```python
from build123d import *

# Parameters (mm, degrees)
SKETCH_1_W          = 25
SKETCH_1_H          = 20
EXTRUDE_1_DEPTH     = 10
EXTRUDE_2_DEPTH     = 10
SKETCH_3_W          = 10
SKETCH_3_H          = 10
CUT_EXTRUDE_1_DEPTH = 15
FILLET_1_DEPTH      = 10
FILLET_START        = -1
FILLET_1_2_DEPTH    = 6
FILLET_1_3_DEPTH    = 6


with BuildPart() as part:
    # 草圖1 → 填料-伸長1 (new body)
    with BuildSketch(Plane(origin=(0, 0, 0), x_dir=(1, 0, 0), z_dir=(0, 1, 0))):
        with Locations((12.5, -10)):
            Rectangle(SKETCH_1_W, SKETCH_1_H)
    extrude(amount=EXTRUDE_1_DEPTH)

    # 草圖2 → 填料-伸長2 (add)
    with BuildSketch(Plane(origin=(0, 10, 0), x_dir=(1, 0, 0), z_dir=(0, 1, 0))):
        Polygon((0, 0), (0, -20), (5, -20), (5, -5), (25, -5), (25, 0), align=None)
    extrude(amount=EXTRUDE_2_DEPTH)

    # 草圖3 → 除料-伸長1 (cut)
    with BuildSketch(Plane.XY.offset(20)):
        with Locations((20, 5)):
            Rectangle(SKETCH_3_W, SKETCH_3_H)
    extrude(amount=-CUT_EXTRUDE_1_DEPTH, mode=Mode.SUBTRACT)

    # 圓角1: read off the stored shape, not the designer's step
    # 圓角1 outline → 圓角1 (add)
    with BuildSketch(Plane(origin=(0, 0, 0), x_dir=(1, 0, 0), z_dir=(0, 1, 0))):
        with BuildLine():
            ThreePointArc((15, -10), (16.464466094, -6.464466094), (20, -5))
            Line((20, -5), (15, -5))
            Line((15, -5), (15, -10))
        make_face()
    extrude(amount=FILLET_1_DEPTH)

    # Fillet 1 2 outline → Fillet 1 2 (cut)
    with BuildSketch(Plane.YZ.offset(FILLET_START)):
        with BuildLine():
            Line((20, 20), (15, 20))
            ThreePointArc((15, 20), (18.535533906, 18.535533906), (20, 15))
            Line((20, 15), (20, 20))
        make_face()
    extrude(amount=FILLET_1_2_DEPTH, mode=Mode.SUBTRACT)

    # Fillet 1 3 outline → Fillet 1 3 (cut)
    with BuildSketch(Plane.XY.offset(FILLET_START)):
        with BuildLine():
            ThreePointArc((20, 20), (23.535533906, 18.535533906), (25, 15))
            Line((25, 15), (25, 20))
            Line((25, 20), (20, 20))
        make_face()
    extrude(amount=FILLET_1_3_DEPTH, mode=Mode.SUBTRACT)


solid = part.part
```
Could you check a few things on this model? Use its own coordinates, in mm. A direction names the side the tool comes from. Coordinates: 2 decimals unless noted, no trailing zeros. Loops run counter-clockwise (first coordinate to the right, second up) from the corner with the lowest first, then second, coordinate; pieces in that order, holes last.
1) Imagine slicing it at A-A (y = 9.25). List the corners of the cut face in (x, z) for me.
Reported:
outline: (0, 0) - (25, 0) - (25, 5) - (20, 5) arc R5 cw to (15, 10) - (15, 20) - (0, 20) - close
2) Please list where these lines run through material, in increasing order: line 1 along X through (y, z) = (11.5, 17); line 2 along X through (y, z) = (8.75, 9.75).
Reported:
line 1: x = 0 to 5
line 2: x = 0 to 15.01
3) Imagine slicing it at C-C (z = 6.75). List the corners of the cut face in (x, y) for me, and give its area (3 significant figures).
Reported:
outline: (0, 0) - (16.2, 0) - (16.2, 10) - (5, 10) - (5, 20) - (0, 20) - close
area: 212 mm2
4) Which directions (+Z, -Z, +X, -X, +Y, -Y) give clear straight access to the entire face, cutting with the end or side of a thin tool? Please do faces 1 (the face through (0, 10, 10)), 2 (the face through (5, 15, 13)), 3 (the face through (15, 5, 15)).
Reported:
face 1: +Z, -Z, -X, +Y, -Y
face 2: +Z, +X, +Y
face 3: +Z, +X, +Y, -Y
5) Imagine slicing it at B-B (x = 17). List the corners of the cut face in (y, z) for me.
Reported:
outline: (0, 0) - (20, 0) - (20, 5) - (10, 5) - (10, 6) - (0, 6) - close
6) Imagine slicing it at D-D (x = 23.75). List the corners of the cut face in (y, z) for me.
Reported:
outline: (0, 0) - (18.31, 0) - (18.31, 5) - (0, 5) - close
7) Will these pins go through, and if not, where does the flat tip stop? pin 1 Ø11 at (y, z) = (7, 16) entering from +X; pin 2 Ø6 at (x, z) = (9, 12) entering from +Y; pin 3 Ø12 at (x, z) = (3, 8.5) entering from -Y; pin 4 Ø8 at (y, z) = (16.5, 15) entering from +X.
Reported:
pin 1: stops at x = 15
pin 2: stops at y = 10
pin 3: stops at y = 0
pin 4: stops at x = 5
